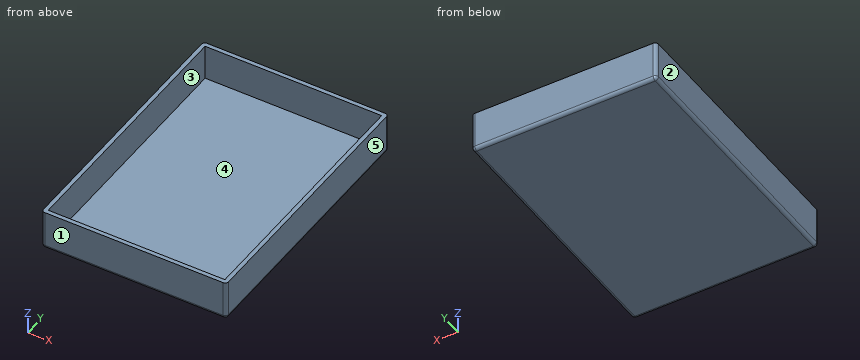
```python
from build123d import *

# Parameters (mm, degrees)
SKETCH1_W           = 88.9
SKETCH1_H           = 127
BOSS_EXTRUDE1_DEPTH = 19.05
FILLET1_R           = 1.5875
SHELL1_T            = -2


with BuildPart() as part:
    # Sketch1 → Boss-Extrude1 (new body)
    with BuildSketch(Plane.XY):
        Rectangle(SKETCH1_W, SKETCH1_H)
    extrude(amount=BOSS_EXTRUDE1_DEPTH)

    # Fillet1
    fillet1_edges = [part.edges().sort_by_distance(p)[0] for p in [
        (-44.45, 0, 0),
        (0, 63.5, 0),
        (44.45, 0, 0),
        (0, -63.5, 0),
        (-44.45, -63.5, 9.525),
        (-44.45, 63.5, 9.525),
        (44.45, 63.5, 9.525),
        (44.45, -63.5, 9.525),
    ]]
    fillet(fillet1_edges, radius=FILLET1_R)

    # Shell1
    shell1_openings = [part.faces().sort_by_distance(p)[0] for p in [
        (0, 0, 19.05),
    ]]
    offset(amount=SHELL1_T, openings=shell1_openings, kind=Kind.INTERSECTION)


solid = part.part
```
Geometry: final body of the model. Coordinates: model frame, mm. Face numbers are marked on the shaded views. A direction names the side the tool comes from. Coordinates: 2 decimals unless noted, no trailing zeros. Answer in a Markdown table with one row per item.
Item 1: Ray query, L1, parallel to X at y = -26, z = 4; L2, parallel to Y at x = -29, z = 2.25; L3, parallel to Z at x = 37.5, y = -45. Return the intervals inside material, ascending.
Return value:
| item | result |
|---|---|
| L1 | x = -44.45 to -42.45, 42.45 to 44.45 |
| L2 | y = -63.5 to -61.5, 61.5 to 63.5 |
| L3 | z = 0 to 2 |
Item 2: Contact query for a flat-ended pin moving along its axis: P1, Ø12, axis at x = 27, y = -15.5, coming from the +Z side. Output: stop coordinate, or through.
Return value:
| item | result |
|---|---|
| P1 | stops at z = 2 |
Item 3: Access query for the marked faces 4 and 5. Directions: +Z, -Z, +X, -X, +Y, -Y. A direction counts if a zero-diameter tool reaches every point of the face in a straight line with its end or side. Return the directions, or none.
Return value:
| item | result |
|---|---|
| face 4 | +Z |
| face 5 | +Z, -Z, +X, +Y, -Y |
Item 4: Draft query along X for the marked faces 1, 2 and 3. Return one class per face: released by +X, released by -X, zero draft, split by the parting line, or undercut.
Return value:
| item | result |
|---|---|
| face 1 | zero draft |
| face 2 | released by -X |
| face 3 | undercut |
